Can you work these out from the model? Positions are in its coordinate system, mm. A direction names the side the tool comes from. Round coordinates to 2 decimals unless told otherwise and drop trailing zeros. Write each loop counter-clockwise with the first axis right and the second up, starting at its lowest first coordinate (ties: lowest second). Pieces come first, ordered by that corner, then holes. Notation, with made-up numbers: M -5,15.5 L 52,15.5 A29 cw 52,44.5 Z; hole C 16.5,12 d1. An arc over 180 degrees is marked long. Answer in a Markdown table with one row per item. Add a question column.
(1) Suppose I cut it at D-D, the plane x = -21. Write out the boundary of the cut face in (y, z).
(2) I'm going to push flat-ended pins straight in: pin 1 (1 mm diameter, centred on y = 9.5, z = 28, fed in from -X); pin 2 (15 mm diameter, centred on x = -270, z = 16, fed in from -Y); pin 3 (8 mm diameter, centred on x = -288, y = -4.5, fed in from +Z); pin 4 (0.6 mm diameter, centred on y = 10, z = 25.5, fed in from +X). Where does each tip first touch, or does it pass through?
(3) For faces 4 (the face through (-163, 15, 15)), 5 (the face through (-161, 11, 26)), 6 (the face through (-161, 0, 15)), which set-ups out of +Z, -Z, +X, -X, +Y, -Y let a thin tool reach every point of the face, with its end or its side?
(4) Suppose I cut it at A-A, the plane y = -12. Write out the boundary of the cut face in (x, z).
(5) If we mould it in two halves opening along X, with no side actions, what happens to faces 1 (the face through (-329, -30, 15)), 2 (the face through (-252, 0, 15)), 3 (the face through (-327.56, 10.07, 15.21))? For each: released by +X, released by -X, zero draft, split by the parting line, or undercut.
(6) If I drill on probe 1 along X at (y, z) = (-1, 28.25); probe 2 along Y at (x, z) = (-198, 22.75); probe 3 along X at (y, z) = (11.5, 3.75), over which ranges is the centre line in solid material (lowest first)?
from build123d import *
from OCP.BRepFilletAPI import BRepFilletAPI_MakeChamfer

# Parameters (mm, degrees)
SKETCH1_W           = 321
SKETCH1_H           = 30
BOSS_EXTRUDE1_DEPTH = 15
SKETCH2_W           = 15
SKETCH2_H           = 30
BOSS_EXTRUDE2_DEPTH = 45
SKETCH3_W           = 40
SKETCH3_H           = 30
BOSS_EXTRUDE3_DEPTH = 0.0001
SKETCH4_W           = 11
SKETCH4_H           = 2
CUT_EXTRUDE1_DEPTH  = 7.2
CHAMFER1_SIZE       = 10
CHAMFER1_SIZE2      = 16.642794824


with BuildPart() as part:
    # Sketch1 → Boss-Extrude1 (new body)
    with BuildSketch(Plane(origin=(0, 0, 0), x_dir=(1, 0, 0), z_dir=(0, 1, 0))):
        with Locations((-160.5, -15)):
            Rectangle(SKETCH1_W, SKETCH1_H)
    extrude(amount=BOSS_EXTRUDE1_DEPTH)

    # Sketch2 → Boss-Extrude2 (add)
    with BuildSketch(Plane(origin=(0, 15, 0), x_dir=(1, 0, 0), z_dir=(0, 1, 0))):
        with Locations((-328.5, -15)):
            Rectangle(SKETCH2_W, SKETCH2_H)
        with Locations((7.5, -15)):
            Rectangle(SKETCH2_W, SKETCH2_H)
    extrude(amount=-BOSS_EXTRUDE2_DEPTH)

    # Sketch3 → Boss-Extrude3 (add)
    with BuildSketch(Plane.XZ):
        with Locations((-160.5, 15)):
            Rectangle(SKETCH3_W, SKETCH3_H)
    extrude(amount=BOSS_EXTRUDE3_DEPTH)

    # Sketch4 → Cut-Extrude1 (cut)
    with BuildSketch(Plane.XY.offset(30)):
        with Locations((-160.5, 10)):
            Rectangle(SKETCH4_W, SKETCH4_H)
    extrude(amount=-CUT_EXTRUDE1_DEPTH, mode=Mode.SUBTRACT)

    # Chamfer1: one chamfer whose edges measure the first distance from different faces: ONE call of the kernel's chamfer builder (chamfer() names one face for all edges)
    chamfer1_edges_1 = [part.edges().sort_by_distance(p)[0] for p in [
        (-336, 15, 15),
    ]]
    chamfer1_side_1 = [part.faces().sort_by_distance(p)[0] for p in [
        (-336, -7.5, 15),
    ]]
    chamfer1_edges_2 = [part.edges().sort_by_distance(p)[0] for p in [
        (15, 15, 15),
    ]]
    chamfer1_side_2 = [part.faces().sort_by_distance(p)[0] for p in [
        (15, -7.5, 15),
    ]]
    chamfer1 = BRepFilletAPI_MakeChamfer(part.part.solid().wrapped)
    for e in chamfer1_edges_1:
        chamfer1.Add(CHAMFER1_SIZE, CHAMFER1_SIZE2, e.wrapped, chamfer1_side_1[0].wrapped)  # the first distance lies on this face
    for e in chamfer1_edges_2:
        chamfer1.Add(CHAMFER1_SIZE, CHAMFER1_SIZE2, e.wrapped, chamfer1_side_2[0].wrapped)  # the first distance lies on this face
    add(Compound.cast(chamfer1.Shape()), mode=Mode.REPLACE)


solid = part.part
Calculated:
| question | item | result |
|---|---|---|
| 1 | outline | M 0,0 L 15,0 L 15,30 L 0,30 Z |
| 2 | pin 1 | x = -329.34 |
| 2 | pin 2 | y = 0 |
| 2 | pin 3 | through |
| 2 | pin 4 | x = 7.18 |
| 3 | face 4 | +Z, -Z, +X, -X, +Y |
| 3 | face 5 | +Z |
| 3 | face 6 | +Z, -Z, -Y |
| 4 | outline | M -336,0 L -321,0 L -321,30 L -336,30 Z; M 0,0 L 15,0 L 15,30 L 0,30 Z |
| 5 | face 1 | zero draft |
| 5 | face 2 | undercut |
| 5 | face 3 | released by -X |
| 6 | probe 1 | -336 to -321, 0 to 15 |
| 6 | probe 2 | 0 to 15 |
| 6 | probe 3 | -325.18 to 4.18 |
